Could you check a few things on this model? Use its own coordinates, in mm. Face numbers are marked on the shaded views. Give positions to 0.01 mm unless a question says otherwise; leave off trailing zeros. Loops run counter-clockwise (first coordinate to the right, second up) from the corner with the lowest first, then second, coordinate; pieces in that order, holes last. Notation, with made-up numbers: (26.25, -17.75) - (73.25, -17.75) arc R17 cw to (73.25, 0.25) - close; hole circle Ø7 at (6.5, -6). An arc over 180 degrees is marked (long way). Write each question's results on one line, items separated by ' | '. Start each with the question number.
(1) Suppose I cut it at A-A (z = -0.25). Please give me the cut outline in (x, y).
(2) I need wall thicknesses on line 1 (Y direction, x = 0, z = 0.75); line 2 (Z direction, x = 0.25, y = 2.5); line 3 (X direction, y = -1, z = 3.25). Which ranges of each line are inside material? Lowest first, please.
(3) Suppose I cut it at B-B (z = -5). Please give me the cut outline in (x, y), and give its area (3 significant figures).
(4) If we mould it in two halves opening along Y, with no side actions, what happens to the marked faces 1, 2 and 3? For each: released by +Y, released by -Y, zero draft, split by the parting line, or undercut.
(5) For pin 1 (3 mm diameter, centred on x = -2, y = -2, fed in from -Z); pin 2 (1.4 mm diameter, centred on x = 0, y = 0, fed in from +Z), each with a flat end and sliding along its axis, tell me the tip position at first contact or that it passes through.
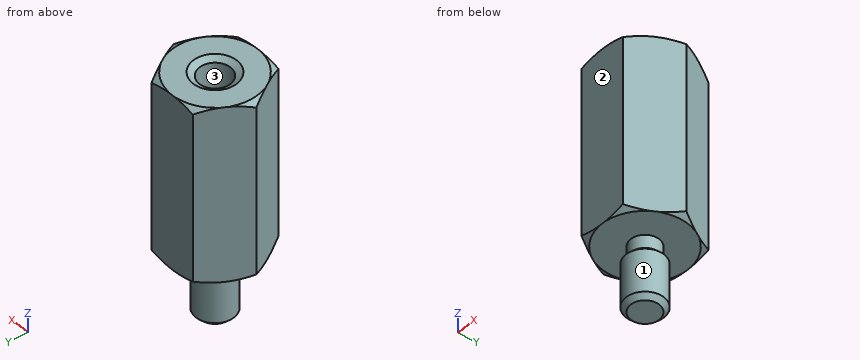
from build123d import *

# Parameters (mm, degrees)
EXTRUDE1_DEPTH                                 = 6.35
F_4_40_TAPPED_HOLE1_STANDARD_DEPTH_D           = 2.2606
F_4_40_TAPPED_HOLE1_STANDARD_DEPTH_DEPTH       = 8.255
F_4_40_TAPPED_HOLE1_STANDARD_DEPTH_CSINK_D     = 3.175
F_4_40_TAPPED_HOLE1_STANDARD_DEPTH_CSINK_ANGLE = 120
F_4_40_TAPPED_HOLE1_STANDARD_DEPTH_TIP         = 0.679152758


with BuildPart() as part:
    # Sketch1 → Extrude1 (new body, symmetric)
    with BuildSketch(Plane.XY):
        Polygon((3.600183074, 0), (1.800091537, 3.11785), (-1.800091537, 3.11785), (-3.600183074, 0), (-1.800091537, -3.11785), (1.800091537, -3.11785), align=None)
    extrude(amount=EXTRUDE1_DEPTH, both=True)

    # Sketch3 → Cut-Revolve1 (revolve, cut)
    with BuildSketch(Plane(origin=(0, 0, 0), x_dir=(0, 0, -1), z_dir=(1, 0, 0))):
        Polygon((-6.35, 3.11785), (-5.47011819, 4.64185), (-6.604, 4.64185), (-6.604, 3.11785), align=None)
    cut_revolve1 = revolve(axis=Axis((0, 0, 6.35), (0, 0, 1)), mode=Mode.SUBTRACT)

    # Mirror1: Cut-Revolve1 across plane
    add(cut_revolve1.mirror(Plane.XY), mode=Mode.SUBTRACT)

    # Sketch2 → 4-40 stud (revolve)
    with BuildSketch(Plane(origin=(0, 0, 0), x_dir=(0, 0, -1), z_dir=(1, 0, 0))):
        Polygon((6.35, 1.03378), (7.3025, 1.03378), (7.648575, 1.379855), (10.766425, 1.379855), (11.1125, 1.03378), (11.1125, 0), (6.35, 0), align=None)
    revolve(axis=Axis((0, 0, -6.35), (0, 0, 1)))

    # #4-40 Tapped Hole1 (STANDARD DEPTH)
    with Locations(Plane.XY.offset(6.35)):
        with Locations((0, 0)):
            CounterSinkHole(F_4_40_TAPPED_HOLE1_STANDARD_DEPTH_D / 2, F_4_40_TAPPED_HOLE1_STANDARD_DEPTH_CSINK_D / 2, depth=F_4_40_TAPPED_HOLE1_STANDARD_DEPTH_DEPTH, counter_sink_angle=F_4_40_TAPPED_HOLE1_STANDARD_DEPTH_CSINK_ANGLE)
            with Locations((0, 0, -(F_4_40_TAPPED_HOLE1_STANDARD_DEPTH_DEPTH + F_4_40_TAPPED_HOLE1_STANDARD_DEPTH_TIP / 2))):  # 118° drill point
                Cone(0, F_4_40_TAPPED_HOLE1_STANDARD_DEPTH_D / 2, F_4_40_TAPPED_HOLE1_STANDARD_DEPTH_TIP, mode=Mode.SUBTRACT)


solid = part.part
Output values:
1) outline: (-3.6, 0) - (-1.8, -3.12) - (1.8, -3.12) - (3.6, 0) - (1.8, 3.12) - (-1.8, 3.12) - close; hole circle Ø2.26 at (0, 0)
2) line 1: -3.12 to -1.13, 1.13 to 3.12 | line 2: -6.35 to 6.35 | line 3: -3.02 to -0.53, 0.53 to 3.02
3) outline: (-3.6, 0) - (-1.8, -3.12) - (1.8, -3.12) - (3.6, 0) - (1.8, 3.12) - (-1.8, 3.12) - close | area: 33.7 mm2
4) face 1: split by the parting line | face 2: released by -Y | face 3: undercut
5) pin 1: z = -10.82 | pin 2: z = -2.16
